Check sheet for the modelled part. Datum: model origin and axes. Units: mm. Give positions to 0.01 mm unless a question says otherwise; leave off trailing zeros. Answer as a JSON object with one key per item and string values.
Autodesk Inventor part; units mm, degrees
ref_plane "工作平面1" through (0, 10, 70) normal (0, 0, 1) x (1, 0, 0)
ref_plane "YZ Plane" through (0, 0, 0) normal (1, 0, 0) x (0, 1, 0)
ref_plane "XZ Plane" through (0, 0, 0) normal (0, 1, 0) x (-1, 0, 0)
sketch "草圖1" plane through (0, 0, 0) normal (1, 0, 0) x (0, 1, 0)
  arc A0 (-14.2857, 20.5163) -> (14.2857, 20.5163) centre (0, 0) ccw
  line L0 (-10, 28.7228) -> (-10, 70)
  line L1 (0, 0) -> (0, 31.1986)
  line L2 (10, 28.7228) -> (10, 70)
  arc A1 (10, 28.7228) -> (14.2857, 20.5163) centre (20, 28.7228) ccw
  arc A2 (-14.2857, 20.5163) -> (-10, 28.7228) centre (-20, 28.7228) ccw
  point P0 (10, 22.9129)
  point P1 (-10, 22.9129)
  dimension "d0" = 50
  dimension "d1" = 20
  dimension "d2" = 10
  dimension "d4" = 70
ref_plane "工作平面1" through (0, 10, 70) normal (0, 0, 1) x (1, 0, 0)
sketch "草圖3" plane through (0, 10, 70) normal (0, 0, 1) x (1, 0, 0)
  circle A0 centre (0, 0) radius 5
  point P0 (0, -10)
  dimension "d3" = 10
sweep "掃掠1" add profiles "草圖3" path "草圖1" path curves L2 A1 A0 A2 L0
properties part number "示範一"
1. Scan lines: L1, parallel to Y at x = 4.5, z = 5; L2, parallel to Z at x = 0, y = 17.5; L3, parallel to Y at x = -1, z = 61. Record each from-to range of solid material in increasing order. Write a range as [from, to].
Determined:
{"L1": "[-26.72, -22.27], [22.27, 26.72]", "L2": "[-24.37, -9.68], [9.68, 24.37]", "L3": "[-14.9, -5.1], [5.1, 14.9]"}
2. Mould release check, pull along Y, two halves, no side actions. Record for faces 1 (the face through (-0.651, 14.957, 49.65)), 2 (the face through (0, 10, 70)): released by +Y, released by -Y, zero draft, split by the parting line, or undercut.
Determined:
{"face 1": "undercut", "face 2": "zero draft"}
3. Go/stop test with flat-tipped pins: P1, Ø3, axis at x = -1.5, y = 22.5, coming from the -Z side; P2, Ø4, axis at y = -14, z = 36, coming from the -X side; P3, Ø4, axis at x = -4, z = 43.5, coming from the +Y side. Record where each tip stops, or that it passes through.
Determined:
{"P1": "z = -21.2", "P2": "x = -4.58", "P3": "y = 14.58"}
